Read the model definition and answer for the solid it produces. Units are mm, in the model's axes. A direction names the side the tool comes from. Coordinates: 2 decimals unless noted, no trailing zeros. Loops run counter-clockwise (first coordinate to the right, second up) from the corner with the lowest first, then second, coordinate; pieces in that order, holes last. Notation, with made-up numbers: M 69.25,32 L 94.25,32 A20 ccw 94.25,61 Z; hole C 62,14.25 d8. An arc over 180 degrees is marked long. One line per item, written item: value. Start each with the question number.
1. The part is cut by section B-B (x = 83). Write down the section's boundary in (y, z).
2. For faces 1 (the face through (-28, 9.752, -2)), 2 (the face through (44.1, -60.1, -2.5)), 3 (the face through (8, -14.248, -2)), determine the directions among +Z, -Z, +X, -X, +Y, -Y from which every point of the face is accessible in a straight line to the end or side of a thin tool.
3. Determine the mould class of faces 4 (the face through (41.7, 10.89, -2.46)), 5 (the face through (68, -61.248, -2)), 6 (the face through (107.01, -10.48, -2.46)), 7 (the face through (19.831, -22, -2)) for opening direction X: +X half, -X half, draft (parallel to the pull), parting line (faces both ways), or undercut.
4. The part is cut by section D-D (y = -52.5). Write down the section's boundary in (x, z).
5. Flat-ended cylindrical pins translate along their axes: pin 1 (3 mm diameter, centred on y = -47, z = -4, fed in from +X); pin 2 (0.9 mm diameter, centred on y = -0.5, z = -2.5, fed in from +X); pin 3 (3 mm diameter, centred on x = 23, z = -2.5, fed in from +Y). Find the tip coordinate at first contact, or state that the pin passes through.
6. The part is cut by section A-A (x = -57). Write down the section's boundary in (y, z), then the cut area to 3 significant figures.
7. Consider probe 1 along Y at (x, z) = (14, -0.6); probe 2 along Y at (x, z) = (67, -4.35); probe 3 along X at (y, z) = (24.5, -3.25). Determine where each line is inside the solid, lowest interval first.
8. The part is cut by section C-C (z = -4.1). State how many separate pieces and enclosed holes the cut face has, then the cut area to 3 significant figures.
```python
from build123d import *

# Parameters (mm, degrees)
ESBO_O1_R             = 1.5
ESBO_O1_R_2           = 1.500000022
ESBO_O1_W             = 5.15
ESBO_O1_H             = 5.150000119
ESBO_O1_H_2           = 10.15
ESBO_O1_H_3           = 8.150000119
ESBO_O1_H_4           = 5.15
FLANGE_BASE1_DEPTH    = 5
ESBO_O2_R             = 1
CORTE_EXTRUS_O1_DEPTH = 5
CORTE_EXTRUS_O2_REACH = 125.402
ESBO_O3_R             = 1.6


# Sheet-metal steps are written as plain solids
with BuildPart() as part:
    # Esboço1 → Flange-base1 (new body)
    with BuildSketch(Plane.XY):
        with BuildLine():
            Line((42.906488073, -57.24787756), (42.906488073, -34.258558753))
            ThreePointArc((42.906488073, -34.258558753), (41.734915199, -31.430131624), (38.906488072, -30.258558747))
            Line((38.906488072, -30.258558747), (-92.146640805, -30.258558747))
            ThreePointArc((-92.146640805, -30.258558747), (-94.975067929, -29.086985872), (-96.146640805, -26.258558747))
            Line((-96.146640805, -26.258558747), (-96.146640805, 5.752123418))
            ThreePointArc((-96.146640805, 5.752123418), (-94.975067929, 8.580550543), (-92.146640805, 9.752123418))
            Line((-92.146640805, 9.752123418), (38.906488017, 9.752123418))
            ThreePointArc((38.906488017, 9.752123418), (41.73491514, 10.923696291), (42.906488017, 13.752123413))
            Line((42.906488017, 13.752123413), (42.906488017, 34.752123929))
            ThreePointArc((42.906488017, 34.752123929), (44.078060914, 37.58055107), (46.906488073, 38.752123924))
            Line((46.906488073, 38.752123924), (87.906488738, 38.752123924))
            ThreePointArc((87.906488738, 38.752123924), (107.013267009, -11.247876821), (87.906488738, -61.247877566))
            Line((87.906488738, -61.247877566), (46.906488073, -61.247877566))
            ThreePointArc((46.906488073, -61.247877566), (44.078060946, -60.076304689), (42.906488073, -57.24787756))
        make_face()
        with Locations((37.406487746, 6.752123154)):
            Circle(ESBO_O1_R, mode=Mode.SUBTRACT)
        with Locations((88.406488193, 19.252123619)):
            Circle(ESBO_O1_R_2, mode=Mode.SUBTRACT)
        with Locations((22.406487746, 6.752123154)):
            Circle(ESBO_O1_R, mode=Mode.SUBTRACT)
        with Locations((7.406487746, 6.752123154)):
            Circle(ESBO_O1_R, mode=Mode.SUBTRACT)
        with Locations((-7.593512254, 6.752123154)):
            Circle(ESBO_O1_R, mode=Mode.SUBTRACT)
        with BuildLine():
            Line((-82.091601362, -6.247877277), (95.906488231, -6.247877277))
            ThreePointArc((95.906488231, -6.247877277), (99.906488003, -10.247877049), (95.906488231, -14.247876821))
            Line((95.906488231, -14.247876821), (-82.093511769, -14.247876821))
            ThreePointArc((-82.093511769, -14.247876821), (-86.093511655, -10.246921617), (-82.091601362, -6.247877277))
        make_face(mode=Mode.SUBTRACT)
        with Locations((37.406490824, 0.252123359)):
            Rectangle(ESBO_O1_W, ESBO_O1_H, mode=Mode.SUBTRACT)
        with Locations((88.406490824, 8.752123299)):
            Rectangle(ESBO_O1_W, ESBO_O1_H_2, mode=Mode.SUBTRACT)
        with Locations((88.406490824, -36.747877)):
            Rectangle(ESBO_O1_W, ESBO_O1_H, mode=Mode.SUBTRACT)
        with Locations((37.406490824, -22.247877)):
            Rectangle(ESBO_O1_W, ESBO_O1_H_3, mode=Mode.SUBTRACT)
        with Locations((88.406490824, 27.252123537)):
            Rectangle(ESBO_O1_W, ESBO_O1_H_4, mode=Mode.SUBTRACT)
        with Locations((22.406490824, 0.252123359)):
            Rectangle(ESBO_O1_W, ESBO_O1_H, mode=Mode.SUBTRACT)
        with Locations((22.406490824, -22.247877)):
            Rectangle(ESBO_O1_W, ESBO_O1_H_3, mode=Mode.SUBTRACT)
        with Locations((7.406490824, 0.252123359)):
            Rectangle(ESBO_O1_W, ESBO_O1_H, mode=Mode.SUBTRACT)
        with Locations((7.406490824, -22.247877)):
            Rectangle(ESBO_O1_W, ESBO_O1_H_3, mode=Mode.SUBTRACT)
        with Locations((-7.593509176, 0.252123359)):
            Rectangle(ESBO_O1_W, ESBO_O1_H, mode=Mode.SUBTRACT)
        with Locations((-7.593509176, -22.247877)):
            Rectangle(ESBO_O1_W, ESBO_O1_H_3, mode=Mode.SUBTRACT)
    extrude(amount=-FLANGE_BASE1_DEPTH)

    # Esboço2 → Corte-extrusão1 (cut)
    with BuildSketch(Plane.XY):
        with Locations((90.981490824, 29.827123537)):
            Circle(ESBO_O2_R)
        with Locations((85.831490824, 29.827123537)):
            Circle(ESBO_O2_R)
        with Locations((85.831490824, 24.677123537)):
            Circle(ESBO_O2_R)
        with Locations((90.981490824, 24.677123537)):
            Circle(ESBO_O2_R)
        with Locations((90.981490824, 13.827123299)):
            Circle(ESBO_O2_R)
        with Locations((85.831490824, 13.827123299)):
            Circle(ESBO_O2_R)
        with Locations((90.981490824, 3.677123299)):
            Circle(ESBO_O2_R)
        with Locations((85.831490824, 3.677123299)):
            Circle(ESBO_O2_R)
        with Locations((85.831490824, -34.17287694)):
            Circle(ESBO_O2_R)
        with Locations((90.981490824, -34.17287694)):
            Circle(ESBO_O2_R)
        with Locations((90.981490824, -39.322877059)):
            Circle(ESBO_O2_R)
        with Locations((85.831490824, -39.322877059)):
            Circle(ESBO_O2_R)
        with Locations((34.831490824, 2.827123418)):
            Circle(ESBO_O2_R)
        with Locations((39.981490824, 2.827123418)):
            Circle(ESBO_O2_R)
        with Locations((39.981490824, -2.322876701)):
            Circle(ESBO_O2_R)
        with Locations((34.831490824, -2.322876701)):
            Circle(ESBO_O2_R)
        with Locations((34.831490824, -18.17287694)):
            Circle(ESBO_O2_R)
        with Locations((39.981490824, -18.17287694)):
            Circle(ESBO_O2_R)
        with Locations((39.981490824, -26.322877059)):
            Circle(ESBO_O2_R)
        with Locations((34.831490824, -26.322877059)):
            Circle(ESBO_O2_R)
        with Locations((19.831490824, 2.827123418)):
            Circle(ESBO_O2_R)
        with Locations((24.981490824, 2.827123418)):
            Circle(ESBO_O2_R)
        with Locations((24.981490824, -2.322876701)):
            Circle(ESBO_O2_R)
        with Locations((19.831490824, -2.322876701)):
            Circle(ESBO_O2_R)
        with Locations((19.831490824, -18.17287694)):
            Circle(ESBO_O2_R)
        with Locations((24.981490824, -18.17287694)):
            Circle(ESBO_O2_R)
        with Locations((24.981490824, -26.322877059)):
            Circle(ESBO_O2_R)
        with Locations((19.831490824, -26.322877059)):
            Circle(ESBO_O2_R)
        with Locations((4.831490824, 2.827123418)):
            Circle(ESBO_O2_R)
        with Locations((9.981490824, 2.827123418)):
            Circle(ESBO_O2_R)
        with Locations((9.981490824, -2.322876701)):
            Circle(ESBO_O2_R)
        with Locations((4.831490824, -2.322876701)):
            Circle(ESBO_O2_R)
        with Locations((4.831490824, -18.17287694)):
            Circle(ESBO_O2_R)
        with Locations((9.981490824, -18.17287694)):
            Circle(ESBO_O2_R)
        with Locations((9.981490824, -26.322877059)):
            Circle(ESBO_O2_R)
        with Locations((4.831490824, -26.322877059)):
            Circle(ESBO_O2_R)
        with Locations((-10.168509176, 2.827123418)):
            Circle(ESBO_O2_R)
        with Locations((-5.018509176, 2.827123418)):
            Circle(ESBO_O2_R)
        with Locations((-5.018509176, -2.322876701)):
            Circle(ESBO_O2_R)
        with Locations((-10.168509176, -2.322876701)):
            Circle(ESBO_O2_R)
        with Locations((-10.168509176, -18.17287694)):
            Circle(ESBO_O2_R)
        with Locations((-5.018509176, -18.17287694)):
            Circle(ESBO_O2_R)
        with Locations((-5.018509176, -26.322877059)):
            Circle(ESBO_O2_R)
        with Locations((-10.168509176, -26.322877059)):
            Circle(ESBO_O2_R)
    extrude(amount=-CORTE_EXTRUS_O1_DEPTH, mode=Mode.SUBTRACT)

    # Esboço3 → Corte-extrusão2 (cut, up to next)
    with BuildSketch(Plane.XY, mode=Mode.PRIVATE) as corte_extrus_o2_sk1:
        with Locations((88.406488193, 19.252123619)):
            Circle(ESBO_O3_R)
    corte_extrus_o2_tool1 = extrude(corte_extrus_o2_sk1.sketch, amount=-CORTE_EXTRUS_O2_REACH, mode=Mode.PRIVATE) & part.part
    # Esboço3 → Corte-extrusão2 (cut, up to next)
    with BuildSketch(Plane.XY, mode=Mode.PRIVATE) as corte_extrus_o2_sk2:
        with Locations((37.406487746, 6.752123154)):
            Circle(ESBO_O3_R)
    corte_extrus_o2_tool2 = extrude(corte_extrus_o2_sk2.sketch, amount=-CORTE_EXTRUS_O2_REACH, mode=Mode.PRIVATE) & part.part
    # Esboço3 → Corte-extrusão2 (cut, up to next)
    with BuildSketch(Plane.XY, mode=Mode.PRIVATE) as corte_extrus_o2_sk3:
        with Locations((22.406487746, 6.752123154)):
            Circle(ESBO_O3_R)
    corte_extrus_o2_tool3 = extrude(corte_extrus_o2_sk3.sketch, amount=-CORTE_EXTRUS_O2_REACH, mode=Mode.PRIVATE) & part.part
    # Esboço3 → Corte-extrusão2 (cut, up to next)
    with BuildSketch(Plane.XY, mode=Mode.PRIVATE) as corte_extrus_o2_sk4:
        with Locations((7.406487746, 6.752123154)):
            Circle(ESBO_O3_R)
    corte_extrus_o2_tool4 = extrude(corte_extrus_o2_sk4.sketch, amount=-CORTE_EXTRUS_O2_REACH, mode=Mode.PRIVATE) & part.part
    # Esboço3 → Corte-extrusão2 (cut, up to next)
    with BuildSketch(Plane.XY, mode=Mode.PRIVATE) as corte_extrus_o2_sk5:
        with Locations((-7.593512254, 6.752123154)):
            Circle(ESBO_O3_R)
    corte_extrus_o2_tool5 = extrude(corte_extrus_o2_sk5.sketch, amount=-CORTE_EXTRUS_O2_REACH, mode=Mode.PRIVATE) & part.part
    add(corte_extrus_o2_tool1.solids().sort_by_distance((88.406488, 19.252124, 0))[0], mode=Mode.SUBTRACT)
    add(corte_extrus_o2_tool2.solids().sort_by_distance((37.406488, 6.752123, 0))[0], mode=Mode.SUBTRACT)
    add(corte_extrus_o2_tool3.solids().sort_by_distance((22.406488, 6.752123, 0))[0], mode=Mode.SUBTRACT)
    add(corte_extrus_o2_tool4.solids().sort_by_distance((7.406488, 6.752123, 0))[0], mode=Mode.SUBTRACT)
    add(corte_extrus_o2_tool5.solids().sort_by_distance((-7.593512, 6.752123, 0))[0], mode=Mode.SUBTRACT)


solid = part.part
```
Answer block:
1. outline: M -61.25,-5 L -14.25,-5 L -14.25,0 L -61.25,0 Z; M -6.25,-5 L 38.75,-5 L 38.75,0 L -6.25,0 Z
2. face 1: +Z, -Z, -X, +Y
2. face 2: +Z, -Z, -X, -Y
2. face 3: +Z, -Z
3. face 4: -X half
3. face 5: draft
3. face 6: +X half
3. face 7: undercut
4. outline: M 42.91,-5 L 94.64,-5 L 94.64,0 L 42.91,0 Z
5. pin 1: stops at x = 98.73
5. pin 2: stops at x = 106.3
5. pin 3: stops at y = 9.75
6. outline: M -30.26,-5 L -14.25,-5 L -14.25,0 L -30.26,0 Z; M -6.25,-5 L 9.75,-5 L 9.75,0 L -6.25,0 Z
6. area: 160 mm2
7. probe 1: y = -30.26 to -14.25, -6.25 to 9.75
7. probe 2: y = -61.25 to -14.25, -6.25 to 38.75
7. probe 3: x = 42.91 to 84.85, 86.82 to 90, 91.97 to 97.94
8. separate pieces: 1
8. enclosed holes: 17
8. area: 9,370 mm2
